Design review of the part built by this model. Coordinates are the model's own, in mm. Face numbers are marked on the shaded views. A direction names the side the tool comes from. Round coordinates to 2 decimals unless told otherwise and drop trailing zeros. Order: outer loops, then holes, each group sorted by start corner. A loop starts at its lowest first (then second) coordinate and runs counter-clockwise, first axis right, second up. Notation, with made-up numbers: (-10.5, 88.5) - (8.5, 88.5) arc R20 ccw to (8.5, 106.5) - close; hole circle Ø1 at (54, -10). An arc over 180 degrees is marked (long way). Use CSV: the item, a comma, the result in double quotes.
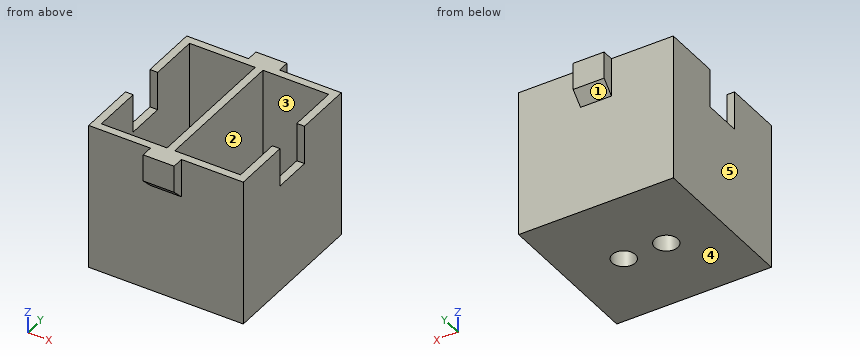
Autodesk Inventor part; units mm, degrees
ref_plane "YZ Plane" through (0, 0, 0) normal (1, 0, 0) x (0, 1, 0)
ref_plane "XZ Plane" through (0, 0, 0) normal (0, 1, 0) x (-1, 0, 0)
ref_plane "XY Plane" through (0, 0, 0) normal (0, 0, 1) x (1, 0, 0)
sketch "Esboço1" plane through (0, 0, 0) normal (0, 0, 1) x (1, 0, 0)
  line L0 (0, 0) -> (20, 0)
  line L1 (20, 0) -> (20, 20)
  line L2 (20, 20) -> (0, 20)
  line L3 (0, 20) -> (0, 0)
  dimension "d0" = 20
  dimension "d1" = 20
extrude "Extrusão1" add sketch "Esboço1" along normal blind 1
sketch "Esboço2" plane through (0, 0, 1) normal (0, 0, 1) x (1, 0, 0)
  circle A0 centre (7.25, 10) radius 1.5
  circle A1 centre (12.75, 10) radius 1.5
  line L0 (0, 0) -> (20, 0)
  line L1 (20, 0) -> (20, 20)
  dimension "d4" = 3
  dimension "d5" = 3
  dimension "d6" = 5.5
  dimension "d7" = 10
  dimension "d8" = 10
  dimension "d9" = 7.25
extrude "Extrusão2" cut sketch "Esboço2" against normal blind 1
sketch "Esboço3" plane through (0, 0, 1) normal (0, 0, 1) x (1, 0, 0)
  circle A0 centre (7.25, 10) radius 1.5
  circle A1 centre (7.25, 10) radius 2
  circle A2 centre (12.75, 10) radius 1.5
  circle A3 centre (12.75, 10) radius 2
  point P0 (0, 0)
  dimension "d12" = 4
  dimension "d13" = 4
extrude "Extrusão3" add sketch "Esboço3" along normal blind 5
sketch "Esboço4" plane through (0, 0, 1) normal (0, 0, 1) x (1, 0, 0)
  line L0 (20, 20) -> (0, 20)
  line L1 (10.5, 20) -> (9.5, 20)
  line L2 (9.5, 20) -> (9.5, 0)
  line L3 (9.5, 0) -> (10.5, 0)
  line L4 (10.5, 0) -> (10.5, 20)
  line L5 (0, 20) -> (0, 0)
  line L6 (20, 0) -> (20, 20)
  line L7 (0, 0) -> (20, 0)
  line L8 (1, 19) -> (19, 19)
  line L9 (19, 19) -> (19, 1)
  line L10 (19, 1) -> (1, 1)
  line L11 (1, 1) -> (1, 19)
  point P0 (9.5, 0)
  point P1 (10.5, 19)
  point P2 (10.5, 1)
  point P3 (9.5, 19)
  point P4 (9.5, 1)
  dimension "d16" = 9.5
  dimension "d17" = 9.5
  dimension "d18" = 0
  dimension "d19" = 1
extrude "Extrusão4" add sketch "Esboço4" along normal blind 18 contours L6 L7 L4 L10 L9 L8 L0 | L4 L8 L2 L0 | L2 L8 L11 L10 L7 L5 L0 | L4 L10 L2 L8 | L3 L2 L10 L4
sketch "Esboço5" plane through (0, 0, 19) normal (0, 0, 1) x (1, 0, 0)
  line L0 (0, 20) -> (0, 0)
  line L1 (1, 1) -> (1, 19)
  line L2 (0, 7.5) -> (1, 7.5)
  line L3 (1, 7.5) -> (1, 12.5)
  line L4 (1, 12.5) -> (0, 12.5)
  line L5 (0, 12.5) -> (0, 7.5)
  line L6 (19, 1) -> (19, 19)
  line L7 (20, 0) -> (20, 20)
  line L8 (19, 7.5) -> (20, 7.5)
  line L9 (20, 7.5) -> (20, 12.5)
  line L10 (20, 12.5) -> (19, 12.5)
  line L11 (19, 12.5) -> (19, 7.5)
  line L12 (20, 20) -> (0, 20)
  point P0 (0, 12.5)
  dimension "d22" = 5
  dimension "d23" = 7.5
  dimension "d24" = 5
  dimension "d25" = 7.5
extrude "Extrusão5" cut sketch "Esboço5" against normal blind 5
sketch "Esboço6" plane through (0, 0, 19) normal (0, 0, 1) x (1, 0, 0)
  line L0 (20, 20) -> (0, 20)
  line L1 (8, 20) -> (12, 20)
  line L2 (12, 20) -> (12, 21.5)
  line L3 (12, 21.5) -> (8, 21.5)
  line L4 (8, 21.5) -> (8, 20)
  line L5 (0, 0) -> (20, 0)
  line L6 (12, 0) -> (8, 0)
  line L7 (8, 0) -> (8, -1.5)
  line L8 (8, -1.5) -> (12, -1.5)
  line L9 (12, -1.5) -> (12, 0)
  dimension "d28" = 8
  dimension "d29" = 8
  dimension "d30" = 1.5
  dimension "d36" = 1.5
  dimension "d37" = 8
  dimension "d38" = 8
extrude "Extrusão6" add sketch "Esboço6" against normal blind 5
chamfer "Chanfro1" distance 1.5 angle 45 2 edges at (10, 21.5, 14) (10, -1.5, 14)
properties part number "caixaled_pt1" material "Plástico PC/ABS"
1) We need section D-D (x = 16). Give the boundary of the cut face in (y, z).
Data:
outline,"(0, 0) - (20, 0) - (20, 19) - (19, 19) - (19, 1) - (1, 1) - (1, 19) - (0, 19) - close"
2) We need section C-C (y = 10.75). Give the boundary of the cut face in (x, z), then the cut area to 3 significant figures.
Data:
outline,"(0, 0) - (5.95, 0) - (5.95, 6) - (5.4, 6) - (5.4, 1) - (1, 1) - (1, 14) - (0, 14) - close; (8.55, 0) - (11.45, 0) - (11.45, 6) - (10.9, 6) - (10.9, 1) - (10.5, 1) - (10.5, 19) - (9.5, 19) - (9.5, 1) - (9.1, 1) - (9.1, 6) - (8.55, 6) - close; (14.05, 0) - (20, 0) - (20, 14) - (19, 14) - (19, 1) - (14.6, 1) - (14.6, 6) - (14.05, 6) - close"
area,"69.9 mm2"
3) We need section B-B (z = 2). Give the boundary of the cut face in (x, y).
Data:
outline,"(0, 0) - (20, 0) - (20, 20) - (0, 20) - close; circle Ø4 at (7.25, 10); circle Ø4 at (12.75, 10); hole (1, 1) - (9.5, 1) - (9.5, 19) - (1, 19) - close; hole circle Ø3 at (7.25, 10); hole (10.5, 1) - (19, 1) - (19, 19) - (10.5, 19) - close; hole circle Ø3 at (12.75, 10)"
4) Insertion check: pin 1 Ø6 at (y, z) = (9.5, 10) entering from -X; pin 2 Ø1.2 at (x, y) = (13.5, 9) entering from +Z; pin 3 Ø0.8 at (x, y) = (0.5, 9.5) entering from +Z; pin 4 Ø1.5 at (x, z) = (4, 10) entering from +Y. Each pin has a flat end and moves straight along its axis. Give the tip position at first contact, or say it passes through.
Data:
pin 1,"stops at x = 0"
pin 2,"stops at z = 6"
pin 3,"stops at z = 14"
pin 4,"stops at y = 20"
5) We need section A-A (x = 7.25). Give the boundary of the cut face in (y, z).
Data:
outline,"(0, 0) - (8.5, 0) - (8.5, 6) - (8, 6) - (8, 1) - (1, 1) - (1, 19) - (0, 19) - close; (11.5, 0) - (20, 0) - (20, 19) - (19, 19) - (19, 1) - (12, 1) - (12, 6) - (11.5, 6) - close"
6) To check wall thickness, follow L1, parallel to X at y = 5.75, z = 15.25; L2, parallel to Y at x = 12.75, z = 1.7; L3, parallel to Y at x = 9, z = 16.25. State the ranges of each line that lie inside material, in increasing order. Write a range as from..to.
Data:
L1,"x = 0..1, 9.5..10.5, 19..20"
L2,"y = 0..1, 8..8.5, 11.5..12, 19..20"
L3,"y = -1.5..1, 19..21.5"
7) For the marked faces 1 and 2, list the 3-axis set-ups (+Z, -Z, +X, -X, +Y, -Y) from which the entire face can be reached by the end or side of a thin tool; tool diameter is ignored.
Data:
face 1,"-Z, +X, -X, +Y"
face 2,"+Z"
8) The part is to be moulded in two halves that separate along X. For the marked faces 3, 4 and 5, say which applies: +X half, -X half, draft (parallel to the pull), parting line (faces both ways), or undercut.
Data:
face 3,"undercut"
face 4,"draft"
face 5,"-X half"
